from build123d import *

# Parameters (mm, degrees)
BOSS_EXTRUDE1_DEPTH = 2
SKETCH5_R           = 2.5
CUT_EXTRUDE1_DEPTH  = 2
SKETCH6_R           = 2.5
CUT_EXTRUDE2_DEPTH  = 2
SKETCH7_R           = 2.5
CUT_EXTRUDE3_DEPTH  = 2
SKETCH8_R           = 2.5
CUT_EXTRUDE4_DEPTH  = 40
SKETCH9_R           = 2.5
CUT_EXTRUDE5_DEPTH  = 40


with BuildPart() as part:
    # Sketch2 → Boss-Extrude1 (new body)
    with BuildSketch(Plane.XY):
        Polygon((47.806423209, 40.776843682), (7.791142002, 66.035659063), (-51.971856858, -28.641512814), (-42.663063156, -46.343104828), (10.441712886, -18.416723725), align=None)
    extrude(amount=BOSS_EXTRUDE1_DEPTH)

    # Sketch5 → Cut-Extrude1 (cut)
    with BuildSketch(Plane.XY.offset(2)):
        with Locations((-11.914275979, -18.874721419)):
            Circle(SKETCH5_R)
    extrude(amount=-CUT_EXTRUDE1_DEPTH, mode=Mode.SUBTRACT)

    # Sketch6 → Cut-Extrude2 (cut)
    with BuildSketch(Plane.XY.offset(2)):
        with Locations((-29.615867993, -28.18351512)):
            Circle(SKETCH6_R)
    extrude(amount=-CUT_EXTRUDE2_DEPTH, mode=Mode.SUBTRACT)

    # Sketch7 → Cut-Extrude3 (cut)
    with BuildSketch(Plane.XY.offset(2)):
        with Locations((7.323304731, -4.622684049)):
            Circle(SKETCH7_R)
    extrude(amount=-CUT_EXTRUDE3_DEPTH, mode=Mode.SUBTRACT)

    # Sketch8 → Cut-Extrude4 (cut)
    with BuildSketch(Plane.XY.offset(2)):
        with Locations((17.998936252, 12.289763781)):
            Circle(SKETCH8_R)
    extrude(amount=-CUT_EXTRUDE4_DEPTH, mode=Mode.SUBTRACT)

    # Sketch9 → Cut-Extrude5 (cut)
    with BuildSketch(Plane.XY.offset(2)):
        with Locations((28.674567773, 29.202211612)):
            Circle(SKETCH9_R)
    extrude(amount=-CUT_EXTRUDE5_DEPTH, mode=Mode.SUBTRACT)


solid = part.part
For this review, take the finished solid that the model builds, in its own axes (mm). Round coordinates to 2 decimals unless told otherwise and drop trailing zeros. Write each loop counter-clockwise with the first axis right and the second up, starting at its lowest first coordinate (ties: lowest second). Pieces come first, ordered by that corner, then holes. Notation, with made-up numbers: M 8.25,-31.75 L 22.25,-31.75 A33 cw 22.25,1.25 Z; hole C 76.5,68.25 d10. An arc over 180 degrees is marked long. Write item = value, one per line. Start each with the question number.
(1) For line 1 along Y through (x, z) = (27.5, 0.1); line 2 along Y through (x, z) = (28, 1.55); line 3 along X through (y, z) = (-30, 0.65), list the stretches that pass through material, from the lowest coordinate up.
(2) We need section A-A (z = 0.4). Give the boundary of the cut face in (x, y), then the cut area to 3 significant figures.
(3) We need section C-C (y = -9.5). Give the boundary of the cut face in (x, z), then the cut area to 3 significant figures.
(4) Clearance check with a flat-ended pin moving along its axis: pin 1 Ø6 at (x, y) = (7.32, -4.62) entering from +Z. State where the tip first meets the part, or that it passes through.
(5) We need section D-D (x = 28.5). Give the boundary of the cut face in (y, z).
(6) The part is to be moulded in two halves that separate along Y. For faces 1 (the face through (-12.24, -16.396, 1.014)), 2 (the face through (28.863, 10.766, 0.986)), 3 (the face through (-3, 11, 0)), say which applies: +Y half, -Y half, draft (parallel to the pull), parting line (faces both ways), or undercut.
(7) We need section B-B (x = -13). Give the boundary of the cut face in (y, z).
Results found:
q1.line_1 = 8.61 to 27, 31.41 to 53.59
q1.line_2 = 9.4 to 26.79, 31.61 to 53.28
q1.line_3 = -51.26 to -31.33, -27.9 to -11.59
q2.outline = M -51.97,-28.64 L -42.66,-46.34 L 10.44,-18.42 L 47.81,40.78 L 7.79,66.04 Z; hole C -29.62,-28.18 d5; hole C -11.91,-18.87 d5; hole C 7.32,-4.62 d5; hole C 18,12.29 d5; hole C 28.67,29.2 d5
q2.area = 4,810 mm²
q3.outline = M -39.89,0 L 16.07,0 L 16.07,2 L -39.89,2 Z
q3.area = 112 mm²
q4.pin_1 = 2
q5.outline = M 10.19,0 L 26.71,0 L 26.71,2 L 10.19,2 Z; M 31.7,0 L 52.96,0 L 52.96,2 L 31.7,2 Z
q6.face_1 = undercut
q6.face_2 = -Y half
q6.face_3 = draft
q7.outline = M -30.74,0 L -21.13,0 L -21.13,2 L -30.74,2 Z; M -16.62,0 L 33.1,0 L 33.1,2 L -16.62,2 Z
